Part model, mm, in its own coordinate system. A direction names the side the tool comes from. Round coordinates to 2 decimals unless told otherwise and drop trailing zeros. Loops run counter-clockwise (first coordinate to the right, second up) from the corner with the lowest first, then second, coordinate; pieces in that order, holes last.
from build123d import *

# Parameters (mm, degrees)
SKETCH1_W           = 100
SKETCH1_H           = 33
BOSS_EXTRUDE1_DEPTH = 5.8
SKETCH2_R           = 3.25
CUT_EXTRUDE1_DEPTH  = 106.463927482
SKETCH3_R           = 6
CUT_EXTRUDE5_DEPTH  = 2.5
FILLET1_R           = 1.5


with BuildPart() as part:
    # Sketch1 → Boss-Extrude1 (new body)
    with BuildSketch(Plane.XY):
        with Locations((50, 16.5)):
            Rectangle(SKETCH1_W, SKETCH1_H)
    extrude(amount=BOSS_EXTRUDE1_DEPTH)

    # Sketch2 → Cut-Extrude1 (cut, through all)
    with BuildSketch(Plane.XY.offset(5.8)):
        with Locations((8, 16.5)):
            Circle(SKETCH2_R)
        with Locations((29, 16.5)):
            Circle(SKETCH2_R)
        with Locations((50, 16.5)):
            Circle(SKETCH2_R)
        with Locations((71, 16.5)):
            Circle(SKETCH2_R)
        with Locations((92, 16.5)):
            Circle(SKETCH2_R)
    extrude(amount=-CUT_EXTRUDE1_DEPTH, mode=Mode.SUBTRACT)

    # Sketch3 → Cut-Extrude5 (cut)
    with BuildSketch(Plane.XY.offset(5.8)):
        with Locations((8, 16.5)):
            Circle(SKETCH3_R)
        with Locations((29, 16.5)):
            Circle(SKETCH3_R)
        with Locations((71, 16.5)):
            Circle(SKETCH3_R)
        with Locations((92, 16.5)):
            Circle(SKETCH3_R)
    extrude(amount=-CUT_EXTRUDE5_DEPTH, mode=Mode.SUBTRACT)

    # Fillet1
    fillet1_edges = [part.edges().sort_by_distance(p)[0] for p in [
        (100, 16.5, 5.8),
        (50, 33, 5.8),
        (0, 16.5, 5.8),
        (50, 33, 0),
        (100, 16.5, 0),
        (50, 0, 0),
        (0, 16.5, 0),
        (0, 33, 2.9),
        (100, 33, 2.9),
        (100, 0, 2.9),
        (0, 0, 2.9),
        (50, 0, 5.8),
    ]]
    fillet(fillet1_edges, radius=FILLET1_R)


solid = part.part
1) Slice it at C-C, the plane y = 21. Give the cut face in (x, z), then the cut area to 3 significant figures.
Values:
outline: (0, 1.5) arc R1.5 ccw to (1.5, 0) - (98.5, 0) arc R1.5 ccw to (100, 1.5) - (100, 4.3) arc R1.5 ccw to (98.5, 5.8) - (95.97, 5.8) - (95.97, 3.3) - (88.03, 3.3) - (88.03, 5.8) - (74.97, 5.8) - (74.97, 3.3) - (67.03, 3.3) - (67.03, 5.8) - (32.97, 5.8) - (32.97, 3.3) - (25.03, 3.3) - (25.03, 5.8) - (11.97, 5.8) - (11.97, 3.3) - (4.03, 3.3) - (4.03, 5.8) - (1.5, 5.8) arc R1.5 ccw to (0, 4.3) - close
area: 499 mm2
2) Drop flat-ended pins along their axis: pin 1 Ø19 at (x, y) = (29, 16.5) entering from +Z; pin 2 Ø5 at (x, y) = (92, 16.5) entering from -Z; pin 3 Ø3.5 at (x, y) = (94, 13.5) entering from +Z. Give the stop position or say it passes through.
Values:
pin 1: stops at z = 5.8
pin 2: passes through
pin 3: stops at z = 3.3
3) Slice it at B-B, the plane x = 50. Give the cut face in (y, z).
Values:
outline: (0, 1.5) arc R1.5 ccw to (1.5, 0) - (13.25, 0) - (13.25, 5.8) - (1.5, 5.8) arc R1.5 ccw to (0, 4.3) - close; (19.75, 0) - (31.5, 0) arc R1.5 ccw to (33, 1.5) - (33, 4.3) arc R1.5 ccw to (31.5, 5.8) - (19.75, 5.8) - close
4) Wall check: line 1 along Y through (x, z) = (8, 2.65); line 2 along Y through (x, z) = (71, 3.9); line 3 along Z through (x, y) = (13.5, 17.5). Give the ranges that are in metal, low to high.
Values:
line 1: y = 0 to 13.25, 19.75 to 33
line 2: y = 0 to 10.5, 22.5 to 33
line 3: z = 0 to 3.3
5) Mould opens along X. For faces 3 (the face through (49, 0, 3)), 4 (the face through (2.006, 16.764, 4.568)), 5 (the face through (100, 16, 3)) say: released by +X, released by -X, zero draft, split by the parting line, or undercut.
Values:
face 3: zero draft
face 4: undercut
face 5: released by +X
6) Tool access for faces 1 (the face through (49, 20, 5.8)), 2 (the face through (86.006, 16.764, 4.568)): list every direction of +Z, -Z, +X, -X, +Y, -Y with a clear straight run to the whole face (end or side of a thin tool).
Values:
face 1: +Z, +X, -X, +Y, -Y
face 2: +Z
7) Slice it at D-D, the plane y = 16.5. Give the number of separate pieces and of enclosed holes in the cut face, then the cut area to 3 significant figures.
Values:
separate pieces: 6
enclosed holes: 0
area: 335 mm2
8) Slice it at A-A, the plane x = 29. Give the cut face in (y, z), then the cut area to 3 significant figures.
Values:
outline: (0, 1.5) arc R1.5 ccw to (1.5, 0) - (13.25, 0) - (13.25, 3.3) - (10.5, 3.3) - (10.5, 5.8) - (1.5, 5.8) arc R1.5 ccw to (0, 4.3) - close; (19.75, 0) - (31.5, 0) arc R1.5 ccw to (33, 1.5) - (33, 4.3) arc R1.5 ccw to (31.5, 5.8) - (22.5, 5.8) - (22.5, 3.3) - (19.75, 3.3) - close
area: 138 mm2
